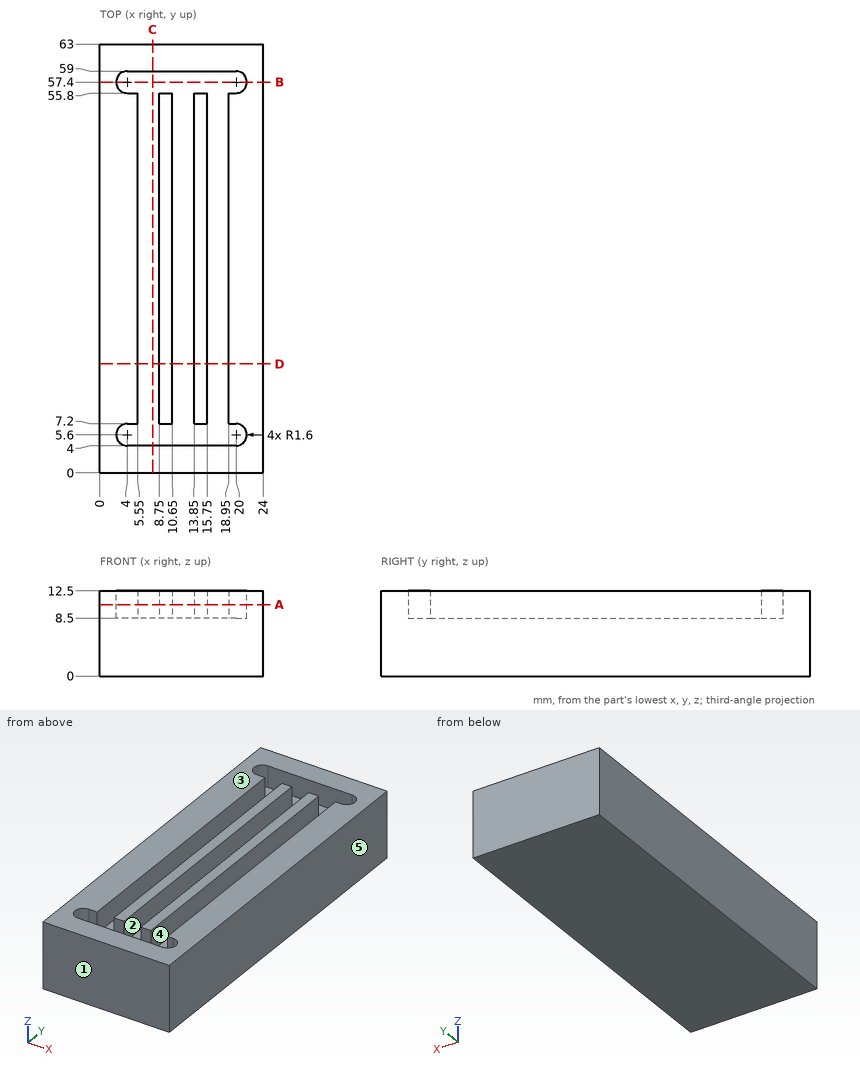
Here's the drawing with two shaded views (mm, measured from the low corner). I have some questions. A direction names the side the tool comes from. Coordinates: 2 decimals unless noted, no trailing zeros. Order: outer loops, then holes, each group sorted by start corner. A loop starts at its lowest first (then second) coordinate and runs counter-clockwise, first axis right, second up. Notation, with made-up numbers: (77, 16) - (120, 16) arc R20 ccw to (120, 35) - close; hole circle Ø9 at (54, 48). An arc over 180 degrees is marked (long way). Answer in a Markdown table with one row per item. Add a question column.
(1) If we section it at B-B, the plane y = 57.4: Please give me the cut outline in (x, z).
(2) If we section it at D-D, the plane y = 16: Please give me the cut outline in (x, z).
(3) If we section it at C-C, the plane x = 7.75: Please give me the cut outline in (y, z).
(4) I need wall thicknesses on L1, parallel to Y at x = 14, z = 9.25; L2, parallel to X at y = 19, z = 11.5; L3, parallel to Y at x = 21, z = 11. Which ranges of each line are inside material? Lowest first, please.
(5) If we section it at A-A, the plane z = 10.5: Please give me the cut outline in (x, y), then the cut area to 3 significant figures.
(6) On a 3-axis mill with a long thin cutter (end or side, diameter ignored), from which of +Z, -Z, +X, -X, +Y, -Y can I reach the whole of each face in a straight line? I mean the marked faces 4 and 5. Say none if no direction works.
(7) Will this pin go through, and if not, where does the flat tip stop? pin 1 (1 mm diameter, centred on x = 14, y = 38.5, fed in from -Z).
(8) If we mould it in two halves opening along Y, with no side actions, what happens to the marked faces 1, 2 and 3? For each: released by +Y, released by -Y, zero draft, split by the parting line, or undercut.
Results are:
| question | item | result |
|---|---|---|
| 1 | outline | (0, 0) - (24, 0) - (24, 12.5) - (21.6, 12.5) - (21.6, 8.5) - (2.4, 8.5) - (2.4, 12.5) - (0, 12.5) - close |
| 2 | outline | (0, 0) - (24, 0) - (24, 12.5) - (18.95, 12.5) - (18.95, 8.5) - (15.75, 8.5) - (15.75, 12.5) - (13.85, 12.5) - (13.85, 8.5) - (10.65, 8.5) - (10.65, 12.5) - (8.75, 12.5) - (8.75, 8.5) - (5.55, 8.5) - (5.55, 12.5) - (0, 12.5) - close |
| 3 | outline | (0, 0) - (63, 0) - (63, 12.5) - (59, 12.5) - (59, 8.5) - (4, 8.5) - (4, 12.5) - (0, 12.5) - close |
| 4 | L1 | y = 0 to 4, 7.2 to 55.8, 59 to 63 |
| 4 | L2 | x = 0 to 5.55, 8.75 to 10.65, 13.85 to 15.75, 18.95 to 24 |
| 4 | L3 | y = 0 to 4.35, 6.85 to 56.15, 58.65 to 63 |
| 5 | outline | (0, 0) - (24, 0) - (24, 63) - (0, 63) - close; (8.75, 7.2) - (10.65, 7.2) - (10.65, 55.8) - (8.75, 55.8) - close; (13.85, 7.2) - (15.75, 7.2) - (15.75, 55.8) - (13.85, 55.8) - close; hole (4, 4) - (20, 4) arc R1.6 ccw to (20, 7.2) - (18.95, 7.2) - (18.95, 55.8) - (20, 55.8) arc R1.6 ccw to (20, 59) - (4, 59) arc R1.6 ccw to (4, 55.8) - (5.55, 55.8) - (5.55, 7.2) - (4, 7.2) arc R1.6 ccw to start |
| 5 | area | 927 mm2 |
| 6 | face 4 | +Z |
| 6 | face 5 | +Z, -Z, +X, +Y, -Y |
| 7 | pin 1 | stops at z = 0 |
| 8 | face 1 | released by -Y |
| 8 | face 2 | undercut |
| 8 | face 3 | zero draft |
